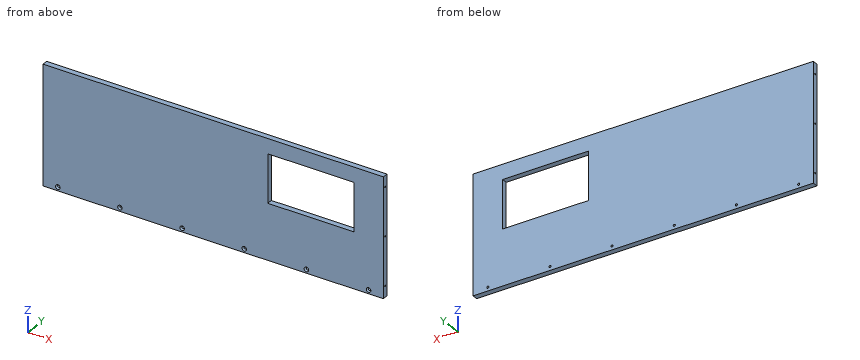
```python
from build123d import *

# Parameters (mm, degrees)
F0_W           = 584.2
F0_H           = 203.2
F1_DEPTH       = 9.525
F3_D           = 3.6576
F3_DEPTH       = 10.3124
F3_CSINK_D     = 7.7978
F3_CSINK_ANGLE = 82
F3_TIP         = 1.0988539001
F4_W           = 147.6502
F4_H           = 82.55
F5_DEPTH       = 9.526
F7_D           = 2.7051
F7_DEPTH       = 13.49375
F7_TIP         = 0.8126940303
F9_D           = 2.7051
F9_DEPTH       = 13.49375
F9_TIP         = 0.8126940303


# Not quite as in the source:
# - a feature names something its author has since deleted; it is built from what else it names


with BuildPart() as f1:
    # F0 (on Front) → F1 (new body)
    with BuildSketch(Plane.XZ):
        with Locations((-292.1, 87.2551402715)):
            Rectangle(F0_W, F0_H)
    extrude(amount=F1_DEPTH)

    # F3
    with Locations(Plane.XZ.offset(9.525)):
        with Locations((-558.8, -7.9948597285), (-345.44, -7.9948597285), (-452.12, -7.9948597285), (-238.76, -7.9948597285), (-132.08, -7.9948597285), (-25.4, -7.9948597285)):
            CounterSinkHole(F3_D / 2, F3_CSINK_D / 2, depth=F3_DEPTH, counter_sink_angle=F3_CSINK_ANGLE)
            with Locations((0, 0, -(F3_DEPTH + F3_TIP / 2))):  # 118° drill point
                Cone(0, F3_D / 2, F3_TIP, mode=Mode.SUBTRACT)

    # F4 (on face) → F5 (cut, through all)
    with BuildSketch(Plane.XZ.offset(9.525)):
        with Locations((-124.6251, 122.1801402715)):
            Rectangle(F4_W, F4_H)
    extrude(amount=-F5_DEPTH, mode=Mode.SUBTRACT)

    # F7
    with Locations(Plane(origin=(-584.2, 0, 0), x_dir=(0, -1, 0), z_dir=(-1, 0, 0))):
        with Locations((4.7625, 169.8051402715), (4.7625, 87.2551402715), (4.7625, 4.7051402715)):
            Hole(F7_D / 2, depth=F7_DEPTH)
            with Locations((0, 0, -(F7_DEPTH + F7_TIP / 2))):  # 118° drill point
                Cone(0, F7_D / 2, F7_TIP, mode=Mode.SUBTRACT)

    # F9
    with Locations(Plane.YZ):
        with Locations((-4.7625, 4.7051402715), (-4.7625, 87.2551402715), (-4.7625, 169.8051402715)):
            Hole(F9_D / 2, depth=F9_DEPTH)
            with Locations((0, 0, -(F9_DEPTH + F9_TIP / 2))):  # 118° drill point
                Cone(0, F9_D / 2, F9_TIP, mode=Mode.SUBTRACT)


solid = f1.part
```
The model under review builds one solid part; all positions refer to its coordinate system, in mm. Round coordinates to 2 decimals unless told otherwise and drop trailing zeros. Order: outer loops, then holes, each group sorted by start corner. A loop starts at its lowest first (then second) coordinate and runs counter-clockwise, first axis right, second up. Notation, with made-up numbers: (37.5, -21) -> (89.5, -21) arc R24 ccw to (89.5, 6) -> close; hole circle Ø2 at (35, -37). An arc over 180 degrees is marked (long way). Use a Markdown table: item, result.
Q1. For line 1 (Z direction, x = -83.5, y = -4); line 2 (X direction, y = -1.25, z = 142.5); line 3 (Z direction, x = -132.08, y = -4.75), list the stretches that pass through material, from the lowest coordinate up.
Values:
| item | result |
|---|---|
| line 1 | z = -14.34 to 80.91, 163.46 to 188.86 |
| line 2 | x = -584.2 to -198.45, -50.8 to 0 |
| line 3 | z = -14.34 to -9.82, -6.17 to 80.91, 163.46 to 188.86 |
Q2. We need section C-C on y = -1.5. Write out the cut boundary in (x, z).
Values:
| item | result |
|---|---|
| outline | (-584.2, -14.34) -> (0, -14.34) -> (0, 188.86) -> (-584.2, 188.86) -> close; hole circle Ø3.66 at (-558.8, -7.99); hole circle Ø3.66 at (-452.12, -7.99); hole circle Ø3.66 at (-345.44, -7.99); hole circle Ø3.66 at (-238.76, -7.99); hole (-198.45, 80.91) -> (-50.8, 80.91) -> (-50.8, 163.46) -> (-198.45, 163.46) -> close; hole circle Ø3.66 at (-132.08, -7.99); hole circle Ø3.66 at (-25.4, -7.99) |
Q3. We need section B-B on x = -73. Write out the cut boundary in (y, z) (3 decimals), then the cut area to 3 significant figures.
Values:
| item | result |
|---|---|
| outline | (-9.525, -14.345) -> (0, -14.345) -> (0, 80.905) -> (-9.525, 80.905) -> close; (-9.525, 163.455) -> (0, 163.455) -> (0, 188.855) -> (-9.525, 188.855) -> close |
| area | 1,150 mm^2 |
Q4. We need section A-A on z = 150.5. Write out the cut boundary in (x, y) (3 decimals).
Values:
| item | result |
|---|---|
| outline | (-584.2, -9.525) -> (-198.45, -9.525) -> (-198.45, 0) -> (-584.2, 0) -> close; (-50.8, -9.525) -> (0, -9.525) -> (0, 0) -> (-50.8, 0) -> close |
Q5. Clearance check with flat-ended pins moving along their axes: P1, Ø2, axis at y = -4.76, z = 4.71, coming from the -X side; P2, Ø2, axis at y = -4.76, z = 169.81, coming from the +X side; P3, Ø2.5, axis at y = -4.76, z = 87.26, coming from the -X side. State where each tip first meets the part, or that it passes through.
Values:
| item | result |
|---|---|
| P1 | stops at x = -570.5 |
| P2 | stops at x = -13.7 |
| P3 | stops at x = -570.65 |
